Geometry check sheet. Reference: the model listing, model coordinates, mm. A direction names the side the tool comes from. Round coordinates to 2 decimals unless told otherwise and drop trailing zeros. Write each loop counter-clockwise with the first axis right and the second up, starting at its lowest first coordinate (ties: lowest second). Pieces come first, ordered by that corner, then holes.
Item 1: Depth check by flat-ended pin: P1, Ø1.5, axis at x = -1.5, z = 2, coming from the -Y side; P2, Ø1.5, axis at x = -1, z = 2, coming from the +Y side; P3, Ø1.5, axis at x = -12.5, z = 1.5, coming from the +Y side. Enter the tip coordinate at first touch or a pass-through.
Item 2: Cross-section at C-C (z = 4.05). Enter the section's corners in (x, y) (3 decimals), then the cut area to 3 significant figures.
Item 3: Scan lines: probe 1 along Y at (x, z) = (0, 3.7) (3 decimals); probe 2 along Z at (x, y) = (5, -17); probe 3 along X at (y, z) = (2.5, 1.85). Record each from-to range of solid material in increasing order.
Item 4: Draft check along Y on faces 4 (the face through (8.767, -16.856, 1.479)), 5 (the face through (-3.2, -2.9, 3)), 6 (the face through (8.2, 4.5, 3)). Enter one of: pulls with the +Y half, pulls with the -Y half, needs draft (parallel to the pull), parting line crosses it, or undercut.
Item 5: Cross-section at A-A (y = 0). Enter the section's corners in (x, z) (3 decimals).
Item 6: Access from +Z, -Z, +X, -X, +Y, -Y to the whole of each face (thin tool, end or side, straight path). Record for faces 1 (the face through (-1.172, 8.923, 4.479)), 2 (the face through (-4.25, 0, 1)), 3 (the face through (4, -2, 6)).
Item 7: Cross-section at D-D (x = -5.5). Enter the section's corners in (y, z), then the cut area to 3 significant figures.
from build123d import *

# Parameters (mm, degrees)
SKETCH_R      = 19
SKETCH_R_2    = 4.125
PAD_DEPTH     = 3
SKETCH001_R   = 9
SKETCH001_R_2 = 4.125
PAD001_DEPTH  = 3
SKETCH002_W   = 8.5
SKETCH002_H   = 8.5
POCKET_DEPTH  = 3


with BuildPart() as part:
    # Sketch → Pad (new body)
    with BuildSketch(Plane.XY):
        Circle(SKETCH_R)
        Circle(SKETCH_R_2, mode=Mode.SUBTRACT)
    extrude(amount=PAD_DEPTH)

    # Sketch001 (on Face4 of Pad) → Pad001 (join)
    with BuildSketch(Plane.XY.offset(3)):
        Circle(SKETCH001_R)
        Circle(SKETCH001_R_2, mode=Mode.SUBTRACT)
    extrude(amount=PAD001_DEPTH)

    # Sketch002 (on Face2 of Pad001) → Pocket (cut)
    with BuildSketch(Plane(origin=(0, 0, 0), x_dir=(1, 0, 0), z_dir=(0, 0, -1))):
        Rectangle(SKETCH002_W, SKETCH002_H)
    extrude(amount=-POCKET_DEPTH, mode=Mode.SUBTRACT)


solid = part.part
Resolved:
1. P1: stops at y = -18.99
1. P2: stops at y = 19
1. P3: stops at y = 14.93
2. outline: circle Ø18 at (0, 0); hole circle Ø8.25 at (0, 0)
2. area: 201 mm2
3. probe 1: y = -9 to -4.125, 4.125 to 9
3. probe 2: z = 0 to 3
3. probe 3: x = -18.83 to -4.25, 4.25 to 18.83
4. face 4: parting line crosses it
4. face 5: undercut
4. face 6: needs draft
5. outline: (-19, 0) - (-4.25, 0) - (-4.25, 3) - (-4.125, 3) - (-4.125, 6) - (-9, 6) - (-9, 3) - (-19, 3) - close; (4.125, 3) - (4.25, 3) - (4.25, 0) - (19, 0) - (19, 3) - (9, 3) - (9, 6) - (4.125, 6) - close
6. face 1: +Z
6. face 2: -Z
6. face 3: +Z, +X, -X, +Y, -Y
7. outline: (-18.19, 0) - (18.19, 0) - (18.19, 3) - (7.12, 3) - (7.12, 6) - (-7.12, 6) - (-7.12, 3) - (-18.19, 3) - close
7. area: 152 mm2
